from build123d import *

# Parameters (mm, degrees)
SKETCH1_W                = 70
SKETCH1_H                = 2
BOSS_EXTRUDE1_DEPTH      = 190.5
BOSS_EXTRUDE2_DEPTH      = 70
SKETCH4_W                = 3
SKETCH4_H                = 29
BOSS_EXTRUDE3_DEPTH      = 44
FILLET1_R                = 40
FILLET2_R                = 10
FILLET3_R                = 5
BOSS_EXTRUDE4_DEPTH      = 15
BOSS_EXTRUDE4_DEPTH_BACK = 15
F_1_4_CLEARANCE_HOLE2_D  = 6.7564
F_1_4_CLEARANCE_HOLE3_D  = 6.7564
M4_CLEARANCE_HOLE1_D     = 4.5
FILLET6_R                = 5
SKETCH23_W               = 29
SKETCH23_H               = 29
CUT_EXTRUDE1_DEPTH       = 2
FILLET7_R                = 5
FILLET8_R                = 5
FILLET9_R                = 5


with BuildPart() as part:
    # Sketch1 → Boss-Extrude1 (new body)
    with BuildSketch(Plane(origin=(0, 0, 0), x_dir=(1, 0, 0), z_dir=(0, 1, 0))):
        Rectangle(SKETCH1_W, SKETCH1_H)
    extrude(amount=BOSS_EXTRUDE1_DEPTH)

    # Sketch3 → Boss-Extrude2 (add)
    with BuildSketch(Plane(origin=(35, 0, 0), x_dir=(0, 0, -1), z_dir=(1, 0, 0))):
        Polygon((1, 0), (-49.2, 0), (1, -25), align=None)
    extrude(amount=-BOSS_EXTRUDE2_DEPTH)

    # Sketch4 → Boss-Extrude3 (add)
    with BuildSketch(Plane.XY.offset(1)):
        with Locations((-26, 163.3)):
            Rectangle(SKETCH4_W, SKETCH4_H)
    extrude(amount=BOSS_EXTRUDE3_DEPTH)

    # Fillet1
    fillet1_edges = [part.edges().sort_by_distance(p)[0] for p in [
        (-26, 148.8, 1),
    ]]
    fillet(fillet1_edges, radius=FILLET1_R)

    # Fillet2
    fillet2_edges = [part.edges().sort_by_distance(p)[0] for p in [
        (-26, 177.8, 1),
    ]]
    fillet(fillet2_edges, radius=FILLET2_R)

    # Fillet3
    fillet3_edges = [part.edges().sort_by_distance(p)[0] for p in [
        (-27.5, 148.3, 1),
    ]]
    fillet(fillet3_edges, radius=FILLET3_R)

    # Sketch9 → Boss-Extrude4 (add, two sides: drawn at the far end of the back side and taken through both)
    with BuildSketch(Plane.ZY.offset(-BOSS_EXTRUDE4_DEPTH_BACK)):
        Polygon((41.249412395, -3.959455979), (41.249412395, -15.459455979), (18.157412395, -15.459455979), align=None)
    extrude(amount=BOSS_EXTRUDE4_DEPTH + BOSS_EXTRUDE4_DEPTH_BACK)

    # 1/4 Clearance Hole2 (through all)
    with Locations(Plane(origin=(0, 0, 0), x_dir=(1, 0, 0), z_dir=(0, 1, 0))):
        with Locations((0, -25.1)):
            Hole(F_1_4_CLEARANCE_HOLE2_D / 2)

    # 1/4 Clearance Hole3 (through all)
    with Locations(Plane(origin=(-24.5, 0, 0), x_dir=(0, 0, -1), z_dir=(1, 0, 0))):
        with Locations((-24.1, 163.3)):
            Hole(F_1_4_CLEARANCE_HOLE3_D / 2)

    # M4 Clearance Hole1 (through all)
    with Locations(Plane.XY.offset(1)):
        with Locations((0, 20), (0, 50), (0, 80), (0, 110)):
            Hole(M4_CLEARANCE_HOLE1_D / 2)

    # Fillet6
    fillet6_edges = [part.edges().sort_by_distance(p)[0] for p in [
        (0, 0, 1),
    ]]
    fillet(fillet6_edges, radius=FILLET6_R)

    # Sketch23 → Cut-Extrude1 (cut)
    with BuildSketch(Plane.XY.offset(1)):
        with Locations((0, 163.3)):
            Rectangle(SKETCH23_W, SKETCH23_H)
    extrude(amount=-CUT_EXTRUDE1_DEPTH, mode=Mode.SUBTRACT)

    # Fillet7
    fillet7_edges = [part.edges().sort_by_distance(p)[0] for p in [
        (-24.5, 148.3, 1),
    ]]
    fillet(fillet7_edges, radius=FILLET7_R)

    # Fillet8
    fillet8_edges = [part.edges().sort_by_distance(p)[0] for p in [
        (35, 190.5, 0),
    ]]
    fillet(fillet8_edges, radius=FILLET8_R)

    # Fillet9
    fillet9_edges = [part.edges().sort_by_distance(p)[0] for p in [
        (-35, 190.5, 0),
    ]]
    fillet(fillet9_edges, radius=FILLET9_R)


solid = part.part
Verification items for the finished model (mm, model axes). A direction names the side the tool comes from. Give positions to 0.01 mm unless a question says otherwise; leave off trailing zeros. Loops run counter-clockwise (first coordinate to the right, second up) from the corner with the lowest first, then second, coordinate; pieces in that order, holes last.
1) Sectioned sample at A-A, the plane y = 163.3. Enter the section's corners in (x, z).
2) Set-up check for faces 4 (the flat face through (0, -10, 41.249)), 5 (the cylindrical face through (-29, 148.85, 2.43)), 6 (the cylindrical face through (-25.49, 131.62, 8.15)): record each of +Z, -Z, +X, -X, +Y, -Y from which the full face is reachable in a straight line by a thin tool's end or side.
3) Draft check along Y on faces 1 (the cylindrical face through (33.57, 189, -0.01)), 2 (the cylindrical face through (0.29, 52.23, -0.01)), 3 (the flat face through (-27.5, 159, 25)). Enter one of: pulls with the +Y half, pulls with the -Y half, needs draft (parallel to the pull), parting line crosses it, or undercut.
4) Sectioned sample at D-D, the plane z = 25.1. Enter the section's corners in (x, y).
5) Sectioned sample at B-B, the plane x = 9. Enter the section's corners in (y, z), then the cut area to 3 significant figures.
6) Thickness scan on line 1 along Y through (x, z) = (0, 0); line 2 along Z through (x, y) = (0, -6); line 3 along Y through (x, z) = (-26.8, 24.1). Record the ranges inside material, lowest first.
7) Sectioned sample at C-C, the plane y = 50. Enter the section's corners in (x, z).
8) Depth check by flat-ended pin: pin 1 Ø3.5 at (x, y) = (-25.5, 166.5) entering from +Z; pin 2 Ø1.5 at (x, y) = (18, 70) entering from +Z; pin 3 Ø1.5 at (x, z) = (13.5, 39) entering from -Y. Enter the tip coordinate at first touch or a pass-through.
Answers:
1. outline: (-35, -1) - (-14.5, -1) - (-14.5, 1) - (-19.5, 1) arc R5 cw to (-24.5, 6) - (-24.5, 20.72) - (-27.5, 20.72) - (-27.5, 6) arc R5 cw to (-32.5, 1) - (-35, 1) - close; (-27.5, 27.48) - (-24.5, 27.48) - (-24.5, 45) - (-27.5, 45) - close; (14.5, -1) - (35, -1) - (35, 1) - (14.5, 1) - close
2. face 4: +Z, +X, -X, -Y
2. face 5: +Z, -X, +Y
2. face 6: +Z, +X, -X
3. face 1: pulls with the +Y half
3. face 2: undercut
3. face 3: needs draft
4. outline: (-35, -12) - (-15, -12) - (-15, -15.46) - (-3.38, -15.46) - (-3.38, 0) - (-35, 0) - close; (-27.5, 145.5) - (-24.5, 145.5) - (-24.5, 160.07) - (-27.5, 160.07) - close; (-27.5, 166.53) - (-24.5, 166.53) - (-24.5, 177.8) - (-27.5, 177.8) - close; (3.38, -15.46) - (15, -15.46) - (15, -12) - (35, -12) - (35, 0) - (3.38, 0) - close
5. outline: (-25, -1) - (148.8, -1) - (148.8, 1) - (5, 1) arc R5 cw to (0, 6) - (0, 49.2) - (-3.96, 41.25) - (-15.46, 41.25) - (-15.46, 18.16) - close; (177.8, -1) - (190.5, -1) - (190.5, 1) - (177.8, 1) - close
5. area: 1,090 mm2
6. line 1: y = -24.5 to 17.75, 22.25 to 47.75, 52.25 to 77.75, 82.25 to 107.75, 112.25 to 148.8, 177.8 to 190.5
6. line 2: z = -1 to 21.72, 28.48 to 41.25
6. line 3: y = -12.5 to 0, 145.05 to 159.92, 166.68 to 177.8
7. outline: (-35, -1) - (-2.25, -1) - (-2.25, 1) - (-35, 1) - close; (2.25, -1) - (35, -1) - (35, 1) - (2.25, 1) - close
8. pin 1: stops at z = 45
8. pin 2: stops at z = 1
8. pin 3: stops at y = -15.46
